```python
from build123d import *

# Parameters (mm, degrees)
BOSS_EXTRUDE1_DEPTH      = 3.175
BOSS_EXTRUDE1_DEPTH_BACK = 1.651


with BuildPart() as part:
    # Sketch1 → Boss-Extrude1 (new, two sides: drawn at the far end of the back side and taken through both)
    with BuildSketch(Plane.XY.offset(-BOSS_EXTRUDE1_DEPTH_BACK)):
        with BuildLine():
            Line((0.8, 5), (23, 5))
            ThreePointArc((23, 5), (28, 0), (23, -5))
            Line((23, -5), (0.8, -5))
            ThreePointArc((0.8, -5), (-4.2, 0), (0.8, 5))
        make_face()
        with BuildLine():
            Line((0, 2), (1, 2))
            ThreePointArc((1, 2), (3, 0), (1, -2))
            Line((1, -2), (0, -2))
            ThreePointArc((0, -2), (-2, 0), (0, 2))
        make_face(mode=Mode.SUBTRACT)
        with BuildLine():
            Line((22.8, 2), (23.8, 2))
            ThreePointArc((23.8, 2), (25.8, 0), (23.8, -2))
            Line((23.8, -2), (22.8, -2))
            ThreePointArc((22.8, -2), (20.8, 0), (22.8, 2))
        make_face(mode=Mode.SUBTRACT)
        with BuildLine():
            Line((18.4, -1), (5.4, -1))
            ThreePointArc((5.4, -1), (4.4, 0), (5.4, 1))
            Line((5.4, 1), (18.4, 1))
            ThreePointArc((18.4, 1), (19.4, 0), (18.4, -1))
        make_face(mode=Mode.SUBTRACT)
    extrude(amount=BOSS_EXTRUDE1_DEPTH + BOSS_EXTRUDE1_DEPTH_BACK)


solid = part.part
```
Here's how the part is built. I have some questions about the finished solid (model axes, mm). A direction names the side the tool comes from. Give positions to 0.01 mm unless a question says otherwise; leave off trailing zeros. Order: outer loops, then holes, each group sorted by start corner. A loop starts at its lowest first (then second) coordinate and runs counter-clockwise, first axis right, second up. Notation, with made-up numbers: M -25.5,19.5 L 14.5,19.5 A21 ccw 14.5,38.5 Z; hole C -29.5,51.25 d2. An arc over 180 degrees is marked long. Use a Markdown table: item, result. Add a question column.
1. Suppose I cut it at D-D (x = 11.5). List the corners of the cut face in (y, z) for me (3 decimals).
2. Suppose I cut it at B-B (y = 0). List the corners of the cut face in (x, z) for me (3 decimals).
3. If we mould it in two halves opening along Y, with no side actions, what happens to faces 3 (the flat face through (12, 5, 1)), 4 (the cylindrical face through (3, 0, 1)), 5 (the flat face through (12.1, 1.2, -1.651)), 6 (the cylindrical face through (-4.2, -0.1, 0.7))? For each: +Y half, -Y half, draft (parallel to the pull), parting line (faces both ways), or undercut.
4. For pin 1 Ø1.5 at (y, z) = (-2, 1.5) entering from +X; pin 2 Ø1 at (y, z) = (-1.5, 1) entering from +X, each with a flat end and sliding along its axis, tell me the tip position at first contact or that it passes through.
5. Suppose I cut it at C-C (z = 0.05). List the corners of the cut face in (x, y) for me.
6. Suppose I cut it at A-A (x = 19). List the corners of the cut face in (y, z) for me (3 decimals).
7. I need wall thicknesses on probe 1 along Y at (x, z) = (11, 1.1); probe 2 along X at (y, z) = (0, 0.9); probe 3 along Y at (x, z) = (5, 2.75). Which ranges of each line are inside material? Lowest first, please. Write a range as from..to.
8. On a 3-axis mill with a long thin cutter (end or side, diameter ignored), from which of +Z, -Z, +X, -X, +Y, -Y can I reach the whole of each face in a straight line? I mean faces 1 (the flat face through (12, -5, 1)), 2 (the flat face through (12, 1, 1)). Say none if no direction works.
Results list:
| question | item | result |
|---|---|---|
| 1 | outline | M -5,-1.651 L -1,-1.651 L -1,3.175 L -5,3.175 Z; M 1,-1.651 L 5,-1.651 L 5,3.175 L 1,3.175 Z |
| 2 | outline | M -4.2,-1.651 L -2,-1.651 L -2,3.175 L -4.2,3.175 Z; M 3,-1.651 L 4.4,-1.651 L 4.4,3.175 L 3,3.175 Z; M 19.4,-1.651 L 20.8,-1.651 L 20.8,3.175 L 19.4,3.175 Z; M 25.8,-1.651 L 28,-1.651 L 28,3.175 L 25.8,3.175 Z |
| 3 | face 3 | +Y half |
| 3 | face 4 | undercut |
| 3 | face 5 | draft |
| 3 | face 6 | parting line |
| 4 | pin 1 | stops at x = 27.84 |
| 4 | pin 2 | stops at x = 27.9 |
| 5 | outline | M 0.8,-5 L 23,-5 A5 ccw 23,5 L 0.8,5 A5 ccw Z; hole M 0,-2 L 1,-2 A2 ccw 1,2 L 0,2 A2 ccw Z; hole M 5.4,-1 L 18.4,-1 A1 ccw 18.4,1 L 5.4,1 A1 ccw Z; hole M 22.8,-2 L 23.8,-2 A2 ccw 23.8,2 L 22.8,2 A2 ccw Z |
| 6 | outline | M -5,-1.651 L -0.8,-1.651 L -0.8,3.175 L -5,3.175 Z; M 0.8,-1.651 L 5,-1.651 L 5,3.175 L 0.8,3.175 Z |
| 7 | probe 1 | y = -5..-1, 1..5 |
| 7 | probe 2 | x = -4.2..-2, 3..4.4, 19.4..20.8, 25.8..28 |
| 7 | probe 3 | y = -5..-0.92, 0.92..5 |
| 8 | face 1 | +Z, -Z, +X, -X, -Y |
| 8 | face 2 | +Z, -Z |
